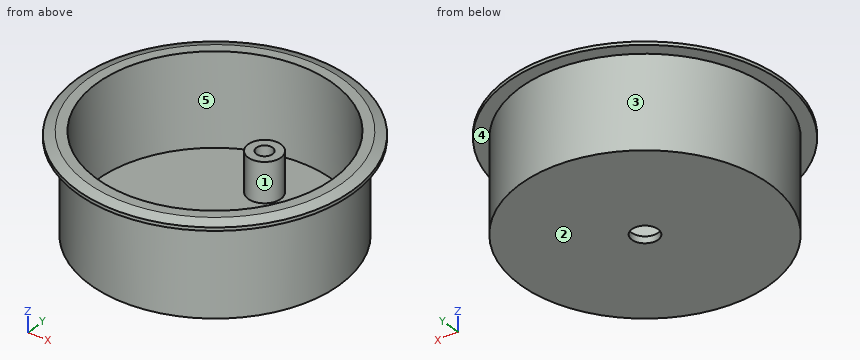
Solid Edge part; units mm, degrees
sketch "Sketch1" plane through (0, 0, 0) normal (0, 0, 1) x (1, 0, 0)
  circle A0 centre (0, 0) radius 19
extrude "Protrusion1" add sketch "Sketch1" along normal blind 1
sketch "Sketch2" plane through (0, 0, 1) normal (0, 0, 1) x (1, 0, 0)
  circle A0 centre (0, 0) radius 19
  circle A1 centre (0, 0) radius 18
extrude "Walls" add sketch "Sketch2" along normal blind 14
sketch "Sketch3" plane through (0, 0, 15) normal (0, 0, 1) x (1, 0, 0)
  circle A0 centre (0, 0) radius 19
  circle A1 centre (0, 0) radius 21
extrude "Top" add sketch "Sketch3" against normal blind 1
sketch "Sketch4" plane through (0, 0, 1) normal (0, 0, 1) x (1, 0, 0)
  circle A0 centre (0, 0) radius 2
extrude "Cutout1" cut sketch "Sketch4" against normal through all
sketch "Sketch5" plane through (0, 0, 1) normal (0, 0, 1) x (1, 0, 0)
  circle A0 centre (0, 10) radius 2.5
extrude "Lock" add sketch "Sketch5" along normal blind 6
hole "Hole___Lock" at (0, 10, 7) direction (0, 0, -1) diameter 2.459 depth 5
chamfer "Chamfer___Top" distance 1.5 distance2 0.5 1 edges at (-21, 0, 15) measured on face at (-14.42, -13.58, 15)
properties material "ABS Plastic, high impact"
Can you work these out from the model? Positions are in its coordinate system, mm. Face numbers are marked on the shaded views. A direction names the side the tool comes from. Round coordinates to 2 decimals unless told otherwise and drop trailing zeros. Loops run counter-clockwise (first coordinate to the right, second up) from the corner with the lowest first, then second, coordinate; pieces in that order, holes last.
Item 1: Suppose I cut it at B-B, the plane z = 5.75. Write out the boundary of the cut face in (x, y).
Item 2: Will these pins go through, and if not, where does the flat tip stop? pin 1 Ø2.5 at (x, y) = (0.5, 10.5) entering from +Z; pin 2 Ø4 at (y, z) = (-0.5, 8.5) entering from +X; pin 3 Ø1.5 at (y, z) = (-6, 5.5) entering from +X; pin 4 Ø3 at (x, y) = (0, 10) entering from -Z.
Item 3: Please list where these lines run through material, in increasing order: L1, parallel to Y at x = 0, z = 3.1; L2, parallel to Y at x = 0, z = 7.5; L3, parallel to Z at x = -7.5, y = 14.
Item 4: Suppose I cut it at C-C, the plane y = 0. Write out the boundary of the cut face in (x, z), then the cut area to 4 significant figures.
Item 5: Suppose I cut it at D-D, the plane z = 1.5. Write out the boundary of the cut face in (x, y).
Item 6: Which directions (+Z, -Z, +X, -X, +Y, -Y) give clear straight access to the entire face, cutting with the end or side of a thin tool? Please do the marked faces 4 and 5.
Item 7: Suppose I cut it at A-A, the plane x = 0. Write out the boundary of the cut face in (y, z).
Item 8: If we mould it in two halves opening along Y, with no side actions, what happens to the marked faces 1, 2 and 3? For each: +Y half, -Y half, draft (parallel to the pull), parting line (faces both ways), or undercut.
Reported:
1. outline: circle Ø38 at (0, 0); circle Ø5 at (0, 10); hole circle Ø36 at (0, 0); hole circle Ø2.46 at (0, 10)
2. pin 1: stops at z = 7
2. pin 2: stops at x = 19
2. pin 3: stops at x = 18.26
2. pin 4: stops at z = 0
3. L1: y = -19 to -18, 7.5 to 8.77, 11.23 to 12.5, 18 to 19
3. L2: y = -19 to -18, 18 to 19
3. L3: z = 0 to 1
4. outline: (-21, 14) - (-19, 14) - (-19, 0) - (-2, 0) - (-2, 1) - (-18, 1) - (-18, 15) - (-19.5, 15) - (-21, 14.5) - close; (2, 0) - (19, 0) - (19, 14) - (21, 14) - (21, 14.5) - (19.5, 15) - (18, 15) - (18, 1) - (2, 1) - close
4. area: 65.25 mm2
5. outline: circle Ø38 at (0, 0); circle Ø5 at (0, 10); hole circle Ø36 at (0, 0)
6. face 4: -Z
6. face 5: +Z
7. outline: (-21, 14) - (-19, 14) - (-19, 0) - (-2, 0) - (-2, 1) - (-18, 1) - (-18, 15) - (-19.5, 15) - (-21, 14.5) - close; (2, 0) - (19, 0) - (19, 14) - (21, 14) - (21, 14.5) - (19.5, 15) - (18, 15) - (18, 1) - (12.5, 1) - (12.5, 7) - (11.23, 7) - (11.23, 2) - (8.77, 2) - (8.77, 7) - (7.5, 7) - (7.5, 1) - (2, 1) - close
8. face 1: undercut
8. face 2: draft
8. face 3: parting line
